from build123d import *

# Parameters (mm, degrees)
SKETCH_1_R               = 32.5
EXTRUDE_1_DEPTH          = 1.5
EXTRUDE_4_DEPTH          = 2
SKETCH_2_R               = 1.75
CUT_EXTRUDE_1_DEPTH      = 7
PATTERN_CIRCULAR_1_COUNT = 3


with BuildPart() as part:
    # 草图1 → 凸台-拉伸1 (new body)
    with BuildSketch(Plane(origin=(0, 0, 0), x_dir=(1, 0, 0), z_dir=(0, 1, 0))):
        with Locations(Location((0, 0, 0), (0, 0, 270))):
            Circle(SKETCH_1_R)
    extrude(amount=EXTRUDE_1_DEPTH)

    # 草图4 → 凸台-拉伸4 (add)
    with BuildSketch(Plane(origin=(0, 1.5, 0), x_dir=(1, 0, 0), z_dir=(0, 1, 0))):
        Polygon((-12.6, 30.722792842), (-12.6, 16.722792842), (12.6, 16.722792842), (12.6, 30.722792842), (10.6, 30.722792842), (10.6, 18.722792842), (-10.6, 18.722792842), (-10.6, 30.722792842), align=None)
    extrude(amount=EXTRUDE_4_DEPTH)

    # 草图2 → 切除-拉伸1 (cut)
    with BuildSketch(Plane.XZ):
        with Locations(Location((0, 24, 0), (0, 0, 270))):
            Circle(SKETCH_2_R)
    cut_extrude_1 = extrude(amount=-CUT_EXTRUDE_1_DEPTH, mode=Mode.SUBTRACT)

    # 阵列(圆周)1: 切除-拉伸1 ×3 about axis
    pattern_circular_1_axis = Axis((0, 0, 0), (0, 1, 0))
    for i in range(1, PATTERN_CIRCULAR_1_COUNT):
        add(cut_extrude_1.rotate(pattern_circular_1_axis, i * 360 / PATTERN_CIRCULAR_1_COUNT), mode=Mode.SUBTRACT)


solid = part.part
Can you work these out from the model? Positions are in its coordinate system, mm. A direction names the side the tool comes from. Round coordinates to 2 decimals unless told otherwise and drop trailing zeros. Order: outer loops, then holes, each group sorted by start corner. A loop starts at its lowest first (then second) coordinate and runs counter-clockwise, first axis right, second up. Notation, with made-up numbers: M -6.5,-20.5 L 38.5,-20.5 A19 ccw 38.5,5.5 Z; hole C 43.5,-9 d7. An arc over 180 degrees is marked long. Use a Markdown table: item, result.
1) Imagine slicing it at C-C (y = 2.8). List the corners of the cut face in (x, z) for me, then the cut area to 3 significant figures.
Geometry says:
| item | result |
|---|---|
| outline | M -12.6,-30.72 L -10.6,-30.72 L -10.6,-18.72 L 10.6,-18.72 L 10.6,-30.72 L 12.6,-30.72 L 12.6,-16.72 L -12.6,-16.72 Z |
| area | 98.4 mm² |
2) Imagine slicing it at A-A (x = 0). List the corners of the cut face in (y, z) for me, then the cut area to 4 significant figures.
Geometry says:
| item | result |
|---|---|
| outline | M 0,-32.5 L 1.5,-32.5 L 1.5,-18.72 L 3.5,-18.72 L 3.5,-16.72 L 1.5,-16.72 L 1.5,22.25 L 0,22.25 Z; M 0,25.75 L 1.5,25.75 L 1.5,32.5 L 0,32.5 Z |
| area | 96.25 mm² |
3) Imagine slicing it at B-B (z = 24). List the corners of the cut face in (x, y) for me, then the cut area to 3 significant figures.
Geometry says:
| item | result |
|---|---|
| outline | M -21.91,0 L -1.75,0 L -1.75,1.5 L -21.91,1.5 Z; M 1.75,0 L 21.91,0 L 21.91,1.5 L 1.75,1.5 Z |
| area | 60.5 mm² |
4) If I drill on line 1 along X through (y, z) = (0.7, -12); line 2 along X through (y, z) = (1.75, -19); line 3 along Z through (x, y) = (-8.5, 2.35), over which ranges is the centre line in solid material (lowest first)?
Geometry says:
| item | result |
|---|---|
| line 1 | x = -30.2 to -22.53, -19.03 to 19.03, 22.53 to 30.2 |
| line 2 | x = -12.6 to -10.6, 10.6 to 12.6 |
| line 3 | z = -18.72 to -16.72 |
5) Imagine slicing it at D-D (x = -8). List the corners of the cut face in (y, z) for me, then the cut area to 3 significant figures.
Geometry says:
| item | result |
|---|---|
| outline | M 0,-31.5 L 1.5,-31.5 L 1.5,-18.72 L 3.5,-18.72 L 3.5,-16.72 L 1.5,-16.72 L 1.5,31.5 L 0,31.5 Z |
| area | 98.5 mm² |
6) I'm going to push flat-ended pins straight in: P1, Ø6, axis at x = -0.5, z = 23.5, coming from the +Y side; P2, Ø1, axis at y = 2.5, z = -24.5, coming from the +X side; P3, Ø1, axis at x = -12, y = 3, coming from the -Z side; P4, Ø5, axis at x = -16.5, z = 22.5, coming from the -Y side. Where does each tip first touch, or does it pass through?
Geometry says:
| item | result |
|---|---|
| P1 | stops at y = 1.5 |
| P2 | stops at x = 12.6 |
| P3 | stops at z = -30.72 |
| P4 | stops at y = 0 |
7) On a 3-axis mill with a long thin cutter (end or side, diameter ignored), from which of +Z, -Z, +X, -X, +Y, -Y can I reach the whole of each face in a straight line? I mean faces 4 (the face through (0, 1.5, -26)), 5 (the face through (-12.6, 2, -24)), 6 (the face through (12.6, 2, -24)). Say none if no direction works.
Geometry says:
| item | result |
|---|---|
| face 4 | -Z, +Y |
| face 5 | +Z, -Z, -X, +Y |
| face 6 | +Z, -Z, +X, +Y |
8) If we mould it in two halves opening along Z, with no side actions, what happens to faces 1 (the face through (0, 0, 0)), 2 (the face through (0.08, 0.74, 25.75)), 3 (the face through (12, 2, -30.723))? For each: +Z half, -Z half, draft (parallel to the pull), parting line (faces both ways), or undercut.
Geometry says:
| item | result |
|---|---|
| face 1 | draft |
| face 2 | undercut |
| face 3 | -Z half |
